Can you work these out from the model? Positions are in its coordinate system, mm. Face numbers are marked on the shaded views. A direction names the side the tool comes from. Round coordinates to 2 decimals unless told otherwise and drop trailing zeros. Order: outer loops, then holes, each group sorted by start corner. A loop starts at its lowest first (then second) coordinate and runs counter-clockwise, first axis right, second up.
Q1. If we section it at D-D (x = 5.5): Please give me the cut outline in (y, z), plus the area to 3 significant figures.
Q2. If we section it at C-C (y = 16.75): Please give me the cut outline in (x, z).
Q3. For the marked faces 1, 2 and 3, which set-ups out of +Z, -Z, +X, -X, +Y, -Y let a thin tool reach every point of the face, with its end or its side?
Q4. Will these pins go through, and if not, where does the flat tip stop? P1, Ø5, axis at x = -11, z = -1, coming from the -Y side; P2, Ø2, axis at x = -11.85, z = 0, coming from the +Y side; P3, Ø1, axis at y = 11.5, z = 0.5, coming from the -X side.
Q5. If we section it at A-A (z = 0): Count the separate pieces of the cut face and the enclosed holes in it, plus the area to 3 significant figures.
Q6. If we section it at B-B (x = 11.5): Please give me the cut outline in (y, z).
Q7. If I drill on line 1 (Z direction, x = 5.5, y = -4.7); line 2 (Y direction, x = 2, z = -3.5); line 3 (X direction, y = 18.25, z = -0.75), over which ranges is the centre line in solid material (lowest first)?
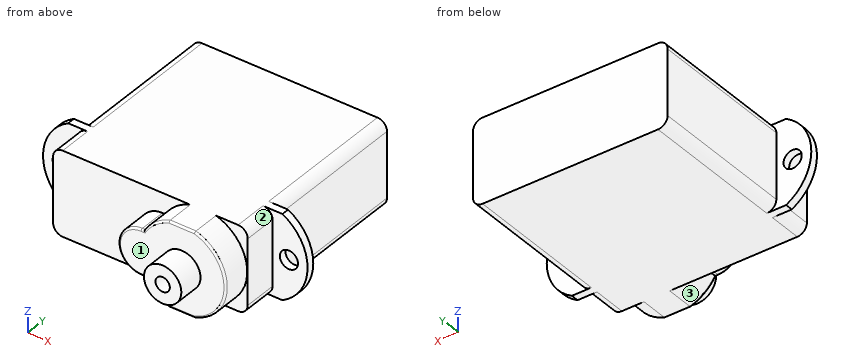
from build123d import *

# Parameters (mm, degrees)
EXTRUDE_1_DEPTH     = 19.6
EXTRUDE_START       = -3.5
EXTRUDE_2_DEPTH     = 0.8
EXTRUDE_3_DEPTH     = 3
FILLET_1_R          = 0.2
SKETCH_4_R          = 1.95
SKETCH_4_R_2        = 0.75
EXTRUDE_4_DEPTH     = 2.7
CUT_EXTRUDE_1_REACH = 18.1
SKETCH_5_R          = 0.95


with BuildPart() as part:
    # Эскиз1 → Бобышка-Вытянуть1 (new body)
    with BuildSketch(Plane(origin=(0, 0, 0), x_dir=(1, 0, 0), z_dir=(0, 1, 0))):
        with BuildLine():
            Line((-9.15, -4.4), (9.15, -4.4))
            ThreePointArc((9.15, -4.4), (9.857106781, -4.107106781), (10.15, -3.4))
            Line((10.15, -3.4), (10.15, 3.4))
            ThreePointArc((10.15, 3.4), (9.857106781, 4.107106781), (9.15, 4.4))
            Line((9.15, 4.4), (-9.15, 4.4))
            ThreePointArc((-9.15, 4.4), (-9.857106781, 4.107106781), (-10.15, 3.4))
            Line((-10.15, 3.4), (-10.15, -3.4))
            ThreePointArc((-10.15, -3.4), (-9.857106781, -4.107106781), (-9.15, -4.4))
        make_face()
    extrude(amount=EXTRUDE_1_DEPTH)

    # Эскиз2 → Бобышка-Вытянуть2 (add)
    with BuildSketch(Plane.XZ.offset(EXTRUDE_START)):
        with BuildLine():
            Line((-9.15, 4.4), (-11.174868417, 4.4))
            ThreePointArc((-11.174868417, 4.4), (-13.8, 0), (-11.174868417, -4.4))
            Line((-11.174868417, -4.4), (-9.15, -4.4))
            ThreePointArc((-9.15, -4.4), (-9.857106781, -4.107106781), (-10.15, -3.4))
            Line((-10.15, -3.4), (-10.15, 3.4))
            ThreePointArc((-10.15, 3.4), (-9.857106781, 4.107106781), (-9.15, 4.4))
        make_face()
        with BuildLine():
            Line((11.174868417, 4.4), (9.15, 4.4))
            ThreePointArc((9.15, 4.4), (9.857106781, 4.107106781), (10.15, 3.4))
            Line((10.15, 3.4), (10.15, -3.4))
            ThreePointArc((10.15, -3.4), (9.857106781, -4.107106781), (9.15, -4.4))
            Line((9.15, -4.4), (11.174868417, -4.4))
            ThreePointArc((11.174868417, -4.4), (13.8, 0), (11.174868417, 4.4))
        make_face()
    extrude(amount=-EXTRUDE_2_DEPTH)

    # Эскиз3 → Бобышка-Вытянуть3 (add)
    with BuildSketch(Plane.XZ):
        with BuildLine():
            ThreePointArc((4.158359214, 4.4), (2.660508694, 3.619017701), (1.545572102, 2.35))
            Line((1.545572102, 2.35), (1.25, 2.35))
            ThreePointArc((1.25, 2.35), (-1.1, 0), (1.25, -2.35))
            Line((1.25, -2.35), (1.545572102, -2.35))
            ThreePointArc((1.545572102, -2.35), (2.660508694, -3.619017701), (4.158359214, -4.4))
            Line((4.158359214, -4.4), (6.841640786, -4.4))
            ThreePointArc((6.841640786, -4.4), (10.1, 0), (6.841640786, 4.4))
            Line((6.841640786, 4.4), (4.158359214, 4.4))
        make_face()
    extrude(amount=EXTRUDE_3_DEPTH)

    # Скругление1
    fillet_1_edges = [part.edges().sort_by_distance(p)[0] for p in [
        (-1.1, -3, 0),
        (2.660508694, -3, -3.619017701),
        (5.5, -3, -4.4),
        (10.1, -3, 0),
        (5.5, -3, 4.4),
        (2.660508694, -3, 3.619017701),
        (1.397786051, -3, -2.35),
        (1.397786051, -3, 2.35),
    ]]
    fillet(fillet_1_edges, radius=FILLET_1_R)

    # Эскиз4 → Бобышка-Вытянуть4 (add)
    with BuildSketch(Plane.XZ.offset(3)):
        with Locations((5.5, 0)):
            Circle(SKETCH_4_R)
        with Locations((5.5, 0)):
            Circle(SKETCH_4_R_2, mode=Mode.SUBTRACT)
    extrude(amount=EXTRUDE_4_DEPTH)

    # Эскиз5 → Вырез-Вытянуть1 (cut, up to next)
    with BuildSketch(Plane.XZ.offset(-3.5), mode=Mode.PRIVATE) as cut_extrude_1_sk1:
        with Locations((-11.85, 0)):
            Circle(SKETCH_5_R)
    cut_extrude_1_tool1 = extrude(cut_extrude_1_sk1.sketch, amount=-CUT_EXTRUDE_1_REACH, mode=Mode.PRIVATE) & part.part
    add(cut_extrude_1_tool1.solids().sort_by_distance((-11.85, 3.5, 0))[0], mode=Mode.SUBTRACT)
    # Эскиз5 → Вырез-Вытянуть1 (cut, up to next)
    with BuildSketch(Plane.XZ.offset(-3.5), mode=Mode.PRIVATE) as cut_extrude_1_sk2:
        with Locations((11.85, 0)):
            Circle(SKETCH_5_R)
    cut_extrude_1_tool2 = extrude(cut_extrude_1_sk2.sketch, amount=-CUT_EXTRUDE_1_REACH, mode=Mode.PRIVATE) & part.part
    add(cut_extrude_1_tool2.solids().sort_by_distance((11.85, 3.5, 0))[0], mode=Mode.SUBTRACT)


solid = part.part
Solution:
1. outline: (-5.7, -1.95) - (-3, -1.95) - (-3, -4.2) arc R0.2 ccw to (-2.8, -4.4) - (19.6, -4.4) - (19.6, 4.4) - (-2.8, 4.4) arc R0.2 ccw to (-3, 4.2) - (-3, 1.95) - (-5.7, 1.95) - (-5.7, 0.75) - (-3, 0.75) - (-3, -0.75) - (-5.7, -0.75) - close
1. area: 205 mm2
2. outline: (-10.15, -3.4) arc R1 ccw to (-9.15, -4.4) - (9.15, -4.4) arc R1 ccw to (10.15, -3.4) - (10.15, 3.4) arc R1 ccw to (9.15, 4.4) - (-9.15, 4.4) arc R1 ccw to (-10.15, 3.4) - close
3. face 1: -Y
3. face 2: +Z, +X, -Y
3. face 3: -Z, -X, -Y
4. P1: stops at y = 0
4. P2: stops at y = 4.3
4. P3: stops at x = -10.15
5. separate pieces: 3
5. enclosed holes: 0
5. area: 441 mm2
6. outline: (3.5, -4.21) - (4.3, -4.21) - (4.3, -0.88) - (3.5, -0.88) - close; (3.5, 0.88) - (4.3, 0.88) - (4.3, 4.21) - (3.5, 4.21) - close
7. line 1: z = -1.95 to -0.75, 0.75 to 1.95
7. line 2: y = 0 to 19.6
7. line 3: x = -10.15 to 10.15
